Print and shaded views of the part. All mm, measured from the part's lowest x, y and z. A direction names the side the tool comes from. Coordinates: 2 decimals unless noted, no trailing zeros. Order: outer loops, then holes, each group sorted by start corner. A loop starts at its lowest first (then second) coordinate and runs counter-clockwise, first axis right, second up. Notation, with made-up numbers: M -4.5,87.5 L 41.5,87.5 A13 ccw 41.5,103.5 Z; hole C 86,6 d11. An arc over 180 degrees is marked long. Return JSON: item names as keys, results as strings.
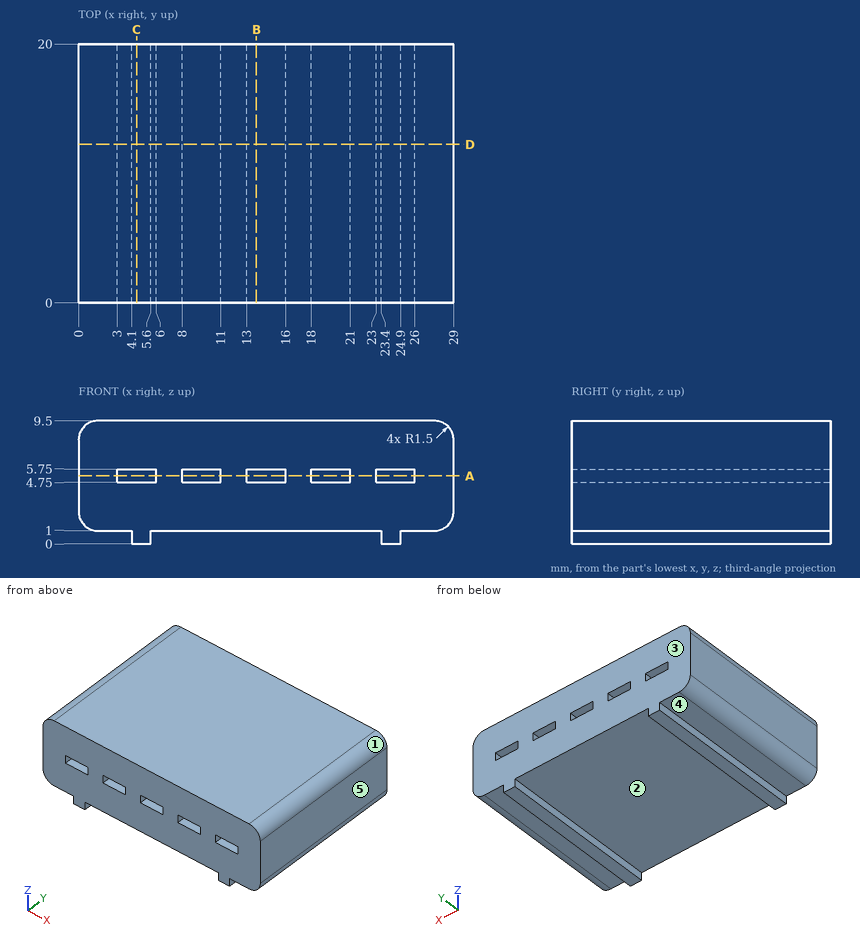
Item 1: Saw through at C-C (x = 4.5). Write the cut outline in (y, z), and give its area (3 significant figures).
Check result:
{"outline": "M 0,0 L 20,0 L 20,4.75 L 0,4.75 Z; M 0,5.75 L 20,5.75 L 20,9.5 L 0,9.5 Z", "area": "170 mm2"}
Item 2: Saw through at D-D (y = 12.25). Count the separate pieces of the cut face and the enclosed holes in it, and give its area (3 significant figures).
Check result:
{"separate pieces": "1", "enclosed holes": "5", "area": "233 mm2"}
Item 3: Saw through at B-B (x = 13.75). Write the cut outline in (y, z).
Check result:
{"outline": "M 0,1 L 20,1 L 20,4.75 L 0,4.75 Z; M 0,5.75 L 20,5.75 L 20,9.5 L 0,9.5 Z"}
Item 4: Pull direction X, two halves, no side cores. Call the marked faces 1, 2 and 3: +X half, -X half, draft (parallel to the pull), parting line (faces both ways), or undercut.
Check result:
{"face 1": "+X half", "face 2": "undercut", "face 3": "draft"}
Item 5: Wall check: line 1 (X direction, y = 15.75, z = 5); line 2 (Z direction, x = 20, y = 18.5); line 3 (X direction, y = 15.25, z = 0.75). Give the ranges that are in metal, low to high.
Check result:
{"line 1": "x = 0 to 3, 6 to 8, 11 to 13, 16 to 18, 21 to 23, 26 to 29", "line 2": "z = 1 to 4.75, 5.75 to 9.5", "line 3": "x = 4.1 to 5.6, 23.4 to 24.9"}
Item 6: Saw through at A-A (z = 5.25). Write the cut outline in (x, y).
Check result:
{"outline": "M 0,0 L 3,0 L 3,20 L 0,20 Z; M 6,0 L 8,0 L 8,20 L 6,20 Z; M 11,0 L 13,0 L 13,20 L 11,20 Z; M 16,0 L 18,0 L 18,20 L 16,20 Z; M 21,0 L 23,0 L 23,20 L 21,20 Z; M 26,0 L 29,0 L 29,20 L 26,20 Z"}
Item 7: 3-axis set-ups, long thin cutter, end or side, ignore diameter. For the marked faces 4 and 5: which of +Z, -Z, +X, -X, +Y, -Y reach the whole face in a straight line?
Check result:
{"face 4": "-Z, -X, +Y, -Y", "face 5": "+Z, -Z, +X, +Y, -Y"}
Item 8: Drop flat-ended pins along their axis: pin 1 Ø0.5 at (y, z) = (14, 0.5) entering from +X; pin 2 Ø1.5 at (x, y) = (10, 6.5) entering from -Z. Give the stop position or say it passes through.
Check result:
{"pin 1": "stops at x = 24.9", "pin 2": "stops at z = 1"}
